```python
from build123d import *

# Parameters (mm, degrees)
EXTRUDE_2_DEPTH    = 8
HOLE_WIZARD_M6_1_D = 5


with BuildPart() as part:
    # 草图1 → 凸台-拉伸2 (new body)
    with BuildSketch(Plane.XY):
        with BuildLine():
            Line((-4, -9.16515139), (-4, -80))
            Line((-4, -80), (4, -80))
            Line((4, -80), (4, -9.16515139))
            ThreePointArc((4, -9.16515139), (0, 10), (-4, -9.16515139))
        make_face()
    extrude(amount=EXTRUDE_2_DEPTH)

    # M6 螺纹孔1 (through all)
    with Locations(Plane.XY.offset(8)):
        with Locations((0, 0)):
            Hole(HOLE_WIZARD_M6_1_D / 2)


solid = part.part
```
Here's how the part is built. I have some questions about the finished solid (model axes, mm). A direction names the side the tool comes from. Give positions to 0.01 mm unless a question says otherwise; leave off trailing zeros. Write each loop counter-clockwise with the first axis right and the second up, starting at its lowest first coordinate (ties: lowest second). Pieces come first, ordered by that corner, then holes. Notation, with made-up numbers: M 78,-6.75 L 100,-6.75 A17 cw 100,19.25 Z; hole C -20,52 d10. An arc over 180 degrees is marked long. Put each result on its own line as item: value. Start each with the question number.
Item 1: If we section it at C-C, the plane z = 2: Write out the boundary of the cut face in (x, y), then the cut area to 3 significant figures.
Item 2: If we section it at B-B, the plane y = 0: Write out the boundary of the cut face in (x, z).
Item 3: I need wall thicknesses on L1, parallel to Y at x = 0, z = 3.5; L2, parallel to X at y = -47.5, z = 4.5; L3, parallel to X at y = 1.5, z = 7. Which ranges of each line are inside material? Lowest first, please. Write a range as from..to.
Item 4: If we section it at D-D, the plane y = -47.5: Write out the boundary of the cut face in (x, z), then the cut area to 3 significant figures.
Item 5: Thinking about a two-plate mould opening in X: for faces 3 (the flat face through (0, -24, 0)), 4 (the cylindrical face through (0, 10, 4)), 5 (the cylindrical face through (0.54, -2.44, 3.94)), 6 (the flat face through (-4, -44, 4)), which applies, +X half, -X half, draft (parallel to the pull), parting line (faces both ways), or undercut?
Item 6: Will these pins go through, and if not, where does the flat tip stop? pin 1 (2 mm diameter, centred on y = -1.5, z = 7, fed in from -X); pin 2 (2 mm diameter, centred on y = -5, z = 6, fed in from +X); pin 3 (2 mm diameter, centred on y = -20.5, z = 6, fed in from -X).
Item 7: On a 3-axis mill with a long thin cutter (end or side, diameter ignored), from which of +Z, -Z, +X, -X, +Y, -Y can I reach the whole of each face in a straight line? I mean faces 1 (the flat face through (4, -45, 4)), 2 (the flat face through (0, -80, 4)). Say none if no direction works.
Item 8: If we section it at A-A, the plane x = 0: Write out the boundary of the cut face in (y, z), then the cut area to 3 significant figures.
Values:
1. outline: M -4,-80 L 4,-80 L 4,-9.17 A10 ccw long -4,-9.17 Z; hole C 0,0 d5
1. area: 857 mm²
2. outline: M -10,0 L -2.5,0 L -2.5,8 L -10,8 Z; M 2.5,0 L 10,0 L 10,8 L 2.5,8 Z
3. L1: -80..-2.5, 2.5..10
3. L2: -4..4
3. L3: -9.89..-2, 2..9.89
4. outline: M -4,0 L 4,0 L 4,8 L -4,8 Z
4. area: 64.0 mm²
5. face 3: draft
5. face 4: parting line
5. face 5: undercut
5. face 6: -X half
6. pin 1: x = -9.99
6. pin 2: x = 9.17
6. pin 3: x = -4
7. face 1: +Z, -Z, +X, -Y
7. face 2: +Z, -Z, +X, -X, -Y
8. outline: M -80,0 L -2.5,0 L -2.5,8 L -80,8 Z; M 2.5,0 L 10,0 L 10,8 L 2.5,8 Z
8. area: 680 mm²
